from build123d import *

# Parameters (mm, degrees)
BOSS_EXTRUDE1_DEPTH      = 10
SKETCH2_W                = 42.944936058
SKETCH2_H                = 25.863004624
SKETCH2_R                = 2.6
BOSS_EXTRUDE2_DEPTH      = 3
SKETCH3_R                = 12.7
BOSS_EXTRUDE5_DEPTH      = 57.47647
BOSS_EXTRUDE4_DEPTH      = 5
BOSS_EXTRUDE4_DEPTH_BACK = 5
SKETCH4_W                = 254
SKETCH4_H                = 330.2
SKETCH4_W_2              = 228.6
SKETCH4_H_2              = 304.8


with BuildPart() as part:
    # Sketch1 → Boss-Extrude1 (new body)
    with BuildSketch(Plane(origin=(0, 0, 0), x_dir=(1, 0, 0), z_dir=(0, 1, 0))):
        Polygon((0, 10), (-8.660254038, 5), (-8.660254038, -5), (0, -10), (8.660254038, -5), (8.660254038, 5), align=None)
    extrude(amount=BOSS_EXTRUDE1_DEPTH)

    # Sketch2 → Boss-Extrude2 (add)
    with BuildSketch(Plane(origin=(0, 10, 0), x_dir=(1, 0, 0), z_dir=(0, 1, 0))):
        Rectangle(SKETCH2_W, SKETCH2_H)
        with Locations(Location((-13.660254038, 0, 0), (0, 0, 270))):
            Circle(SKETCH2_R, mode=Mode.SUBTRACT)
        with Locations(Location((13.660254038, 0, 0), (0, 0, 90))):
            Circle(SKETCH2_R, mode=Mode.SUBTRACT)
    extrude(amount=BOSS_EXTRUDE2_DEPTH)

    # Sketch3 → Boss-Extrude5 (add)
    with BuildSketch(Plane(origin=(0, 13, 0), x_dir=(1, 0, 0), z_dir=(0, 1, 0))):
        with Locations(Location((0, 0, 0), (0, 0, 10.525215122))):
            Circle(SKETCH3_R)
    extrude(amount=BOSS_EXTRUDE5_DEPTH)

    # Sketch4 → Boss-Extrude4 (add, two sides: drawn at the far end of the back side and taken through both)
    with BuildSketch(Plane.XY.offset(-BOSS_EXTRUDE4_DEPTH_BACK)):
        with Locations((0, 235.57647)):
            Rectangle(SKETCH4_W, SKETCH4_H)
        with Locations((0, 235.57647)):
            Rectangle(SKETCH4_W_2, SKETCH4_H_2, mode=Mode.SUBTRACT)
    extrude(amount=BOSS_EXTRUDE4_DEPTH + BOSS_EXTRUDE4_DEPTH_BACK)


solid = part.part
Geometry: final body of the model. Coordinates: model frame, mm. A direction names the side the tool comes from. Round coordinates to 2 decimals unless told otherwise and drop trailing zeros. Loops run counter-clockwise (first coordinate to the right, second up) from the corner with the lowest first, then second, coordinate; pieces in that order, holes last. Notation, with made-up numbers: M 19.25,68.25 L 64.25,68.25 A24 ccw 64.25,90.25 Z; hole C 34.25,86.25 d6. An arc over 180 degrees is marked long. Put each result on its own line as item: value. Start each with the question number.
(1) Section query B-B (x = 92). Return loops of the section in (y, z).
(2) Material intervals for line 1 along X through (y, z) = (11.2, 0); line 2 along Y through (x, z) = (-62, 1.75); line 3 along X through (y, z) = (115, 0), sorted ascending. Write a range as [from, to].
(3) Contact query for flat-ended pins moving along their axis: pin 1 Ø4 at (x, z) = (1.5, 10) entering from +Y; pin 2 Ø0.8 at (x, z) = (12, 0.5) entering from -Y; pin 3 Ø3 at (y, z) = (3.5, 1) entering from -X. Output: stop coordinate, or through.
(4) Draft query along Y for faces 1 (the face through (114.3, 233, 0)), 2 (the face through (-4.27, 4.93, -7.535)), 3 (the face through (9, 10, 0)). Return one class per face: +Y half, -Y half, draft (parallel to the pull), parting line (faces both ways), or undercut.
(5) Section query A-A (y = 120). Return loops of the section in (x, z).
(6) Set-up query: faces 4 (the face through (-10.77, 41.34, -6.73)), 5 (the face through (8.66, 5, 0)), 6 (the face through (-2, 83.176, 0)). Return all of +Z, -Z, +X, -X, +Y, -Y with unobstructed straight access to the full face (end or side cutting, diameter ignored); none if empty.
Findings below:
1. outline: M 70.48,-5 L 83.18,-5 L 83.18,5 L 70.48,5 Z; M 387.98,-5 L 400.68,-5 L 400.68,5 L 387.98,5 Z
2. line 1: x = [-21.47, -16.26], [-11.06, 11.06], [16.26, 21.47]
2. line 2: y = [70.48, 83.18], [387.98, 400.68]
2. line 3: x = [-127, -114.3], [114.3, 127]
3. pin 1: stops at y = 70.48
3. pin 2: stops at y = 13
3. pin 3: stops at x = -8.66
4. face 1: undercut
4. face 2: draft
4. face 3: -Y half
5. outline: M -127,-5 L -114.3,-5 L -114.3,5 L -127,5 Z; M 114.3,-5 L 127,-5 L 127,5 L 114.3,5 Z
6. face 4: none
6. face 5: +Z, -Z, +X, -Y
6. face 6: +Z, -Z
